Check sheet for the modelled part. Datum: model origin and axes. Units: mm. A direction names the side the tool comes from. Coordinates: 2 decimals unless noted, no trailing zeros. Loops run counter-clockwise (first coordinate to the right, second up) from the corner with the lowest first, then second, coordinate; pieces in that order, holes last. Notation, with made-up numbers: M -30,-21.5 L 5,-21.5 A30 ccw 5,1.5 Z; hole C -23.75,76 d5. An arc over 180 degrees is marked long. Return JSON: item names as keys, results as strings.
Autodesk Inventor part; units mm, degrees
ref_plane "YZ Plane" through (0, 0, 0) normal (1, 0, 0) x (0, 1, 0)
ref_plane "XZ Plane" through (0, 0, 0) normal (0, 1, 0) x (-1, 0, 0)
ref_plane "XY Plane" through (0, 0, 0) normal (0, 0, 1) x (1, 0, 0)
ref_plane "Work Plane1" through (0, 0, 0) normal (0, 0, 1) x (1, 0, 0)
sketch "Sketch1" plane through (0, 0, 0) normal (0, 0, 1) x (1, 0, 0)
  circle A0 centre (-32.16, 25) radius 1.5
  line L0 (-46.16, -18.25) -> (4.84, -18.25)
  line L1 (4.84, -18.25) -> (4.84, 0.75)
  line L2 (4.84, 0.75) -> (-46.16, 0.75)
  line L3 (-46.16, -18.25) -> (-46.16, 0.75)
  line L4 (4.84, 68.25) -> (-46.16, 68.25)
  line L5 (-46.16, 68.25) -> (-46.16, 49.25)
  line L6 (-46.16, 49.25) -> (4.84, 49.25)
  line L7 (4.84, 68.25) -> (4.84, 49.25)
  line L8 (-37.16, 68.25) -> (-27.16, 68.25)
  line L9 (-27.16, 68.25) -> (-27.16, -18.25)
  line L10 (-27.16, -18.25) -> (-37.16, -18.25)
  line L11 (-37.16, -18.25) -> (-37.16, 68.25)
  line L12 (-37.16, 68.25) -> (-27.16, -18.25) construction
  line L13 (-27.16, 68.25) -> (-37.16, -18.25) construction
  point P0 (0, 0)
  dimension "d0" = 10
ref_plane "Work Plane3" through (-27.16, 68.25, 0) normal (1, 0, 0) x (0, -1, 0)
ref_plane "Work Plane2" through (4.84, 54, -29.8) normal (1, 0, 0) x (0, -1, 0)
sketch "Sketch2" plane through (-27.16, 68.25, 0) normal (1, 0, 0) x (0, -1, 0)
  line L0 (58.4964, 22.9) -> (28.0036, 22.9)
  line L1 (65, 22.8) -> (65, 15.8)
  line L2 (86.7048, 0.0852) -> (64.4463, 0.0852)
  line L3 (64.4463, 0.0852) -> (64.4463, -2.9148)
  line L4 (64.4463, -2.9148) -> (86.7048, -2.9148)
  line L5 (86.7048, -2.9148) -> (86.7048, 0.0852)
  line L6 (43.25, 22.9) -> (52.25, 22.9)
  line L7 (52.25, 22.9) -> (52.25, 18.9)
  line L8 (52.25, 18.9) -> (43.25, 18.9)
  line L9 (43.25, 18.9) -> (43.25, 22.9)
  line L10 (64.4463, 0.0852) -> (52.25, 22.9)
  line L11 (50.14, 18.9) -> (64.0461, -2.9148)
  line L12 (64.0461, -2.9148) -> (64.4463, -2.9148)
  point P0 (68.25, 0)
  dimension "d1" = 3
  dimension "d2" = 9
  dimension "d3" = 4
extrude "Extrusion1" add sketch "Sketch2" against normal blind 10
mirror "Mirror1" about plane through (-27.16, 25, -18.9) normal (0, 1, 0) of "Extrusion1"
sketch "Sketch3" plane through (-37.16, 18.11, -18.9) normal (0, 0, 1) x (1, 0, 0)
  circle A0 centre (5, 6.89) radius 1.5
  point P0 (37.16, -18.11)
hole "Hole1" at (-32.16, 25, -18.9) direction (0, 0, -1) diameter 3 end through all counterbore diameter 7 counterbore depth 0.5
move faces "Move1" translate (3, 0, 0) faces at (-27.16, 37.3621, -13.9617)
fillet "Fillet1" radius 4 6 edges at (-30.66, 31.89, -18.9) (-30.66, 18.11, -18.9) (-30.66, 3.8037, -0.0852) (-30.66, 46.1963, -0.0852) (-30.66, 45.7961, 2.9148) (-30.66, 4.2039, 2.9148)
properties part number "servo_bracket_holder"
1) Go/stop test with flat-tipped pins: pin 1 Ø1.5 at (x, y) = (-31.5, -3.5) entering from -Z; pin 2 Ø4 at (x, y) = (-32.5, 47) entering from +Z; pin 3 Ø5.5 at (x, y) = (-30.5, 26.5) entering from +Z; pin 4 Ø6 at (y, z) = (12, 0) entering from -X. Record where each tip stops, or that it passes through.
Answers:
{"pin 1": "z = -0.09", "pin 2": "z = 2.91", "pin 3": "z = -18.9", "pin 4": "through"}
2) Section check A-A on y = 25. Record the cut outline in (x, z).
Answers:
{"outline": "M -37.16,-22.9 L -33.66,-22.9 L -33.66,-19.4 L -35.66,-19.4 L -35.66,-18.9 L -37.16,-18.9 Z; M -30.66,-22.9 L -24.16,-22.9 L -24.16,-18.9 L -28.66,-18.9 L -28.66,-19.4 L -30.66,-19.4 Z"}
3) Draft check along Y on faces 5 (the face through (-30.57, 31.6, -18.42)), 6 (the face through (-31, -8, 2.915)), 7 (the face through (-31, 68.455, 1)). Enter one of: +Y half, -Y half, draft (parallel to the pull), parting line (faces both ways), or undercut.
Answers:
{"face 5": "undercut", "face 6": "draft", "face 7": "+Y half"}
4) Set-up check for faces 1 (the face through (-30.57, 11.24, -8.12)), 2 (the face through (-31, -9, -0.085)), 3 (the face through (-35.63, 25.46, -19.15)), 4 (the face through (-30.696, 25.325, -21.174)): record each of +Z, -Z, +X, -X, +Y, -Y from which the full face is reachable in a straight line by a thin tool's end or side.
Answers:
{"face 1": "+Z, +X, -X", "face 2": "-Z, +X, -X, -Y", "face 3": "+Z", "face 4": "+Z, -Z"}
5) Section check D-D on x = -27.25. Record the cut outline in (y, z).
Answers:
{"outline": "M -18.45,-0.09 L 1.41,-0.09 A4 cw 4.93,-2.2 L 16,-22.9 L 34,-22.9 L 45.07,-2.2 A4 cw 48.59,-0.09 L 68.45,-0.09 L 68.45,2.91 L 47.99,2.91 A4 ccw 44.62,1.06 L 33.07,-17.05 A4 cw 29.7,-18.9 L 20.3,-18.9 A4 cw 16.93,-17.05 L 5.38,1.06 A4 ccw 2.01,2.91 L -18.45,2.91 Z"}
6) Scan lines: line 1 along X through (y, z) = (25, -18.95); line 2 along X through (y, z) = (25, -20.4); line 3 along Z through (x, y) = (-27.25, 28). Record each from-to range of solid material in increasing order. Write a range as [from, to].
Answers:
{"line 1": "[-37.16, -35.66], [-28.66, -24.16]", "line 2": "[-37.16, -33.66], [-30.66, -24.16]", "line 3": "[-22.9, -18.9]"}
7) Section check C-C on z = -10. Record the cut outline in (x, y).
Answers:
{"outline": "M -37.16,9.1 L -24.16,9.1 L -24.16,12.44 L -37.16,12.44 Z; M -37.16,37.56 L -24.16,37.56 L -24.16,40.9 L -37.16,40.9 Z"}
8) Section check B-B on x = -32.16. Record the cut outline in (y, z), then the cut area to 3 significant figures.
Answers:
{"outline": "M -18.45,-0.09 L 1.41,-0.09 A4 cw 4.93,-2.2 L 16,-22.9 L 23.5,-22.9 L 23.5,-19.4 L 21.5,-19.4 L 21.5,-18.9 L 20.3,-18.9 A4 cw 16.93,-17.05 L 5.38,1.06 A4 ccw 2.01,2.91 L -18.45,2.91 Z; M 26.5,-22.9 L 34,-22.9 L 45.07,-2.2 A4 cw 48.59,-0.09 L 68.45,-0.09 L 68.45,2.91 L 47.99,2.91 A4 ccw 44.62,1.06 L 33.07,-17.05 A4 cw 29.7,-18.9 L 28.5,-18.9 L 28.5,-19.4 L 26.5,-19.4 Z", "area": "334 mm²"}
